Work out the finished part from the listing and answer in its coordinate system (mm). A direction names the side the tool comes from. Round coordinates to 2 decimals unless told otherwise and drop trailing zeros. Write each loop counter-clockwise with the first axis right and the second up, starting at its lowest first coordinate (ties: lowest second). Pieces come first, ordered by that corner, then holes.
from build123d import *

# Parameters (mm, degrees)
SKETCH_1_R          = 10
SKETCH_1_R_2        = 6
EXTRUDE_2_DEPTH     = 13
SKETCH_2_OUTSIDE_W  = 28.226
SKETCH_2_OUTSIDE_H  = 28.226
SKETCH_2_OUTSIDE_R  = 8.5
CUT_EXTRUDE_1_DEPTH = 9
CHAMFER_1_SIZE      = 0.5


with BuildPart() as part:
    # 草图1 → 凸台-拉伸2 (new body)
    with BuildSketch(Plane(origin=(0, 0, 0), x_dir=(0, 0, -1), z_dir=(1, 0, 0))):
        with Locations(Location((0, 0, 0), (0, 0, 180))):
            Circle(SKETCH_1_R)
        with Locations(Location((0, 0, 0), (0, 0, 180))):
            Circle(SKETCH_1_R_2, mode=Mode.SUBTRACT)
    extrude(amount=EXTRUDE_2_DEPTH)

    # 草图2 outside → 切除-拉伸1 (cut)
    with BuildSketch(Plane(origin=(13, 0, 0), x_dir=(0, 0, -1), z_dir=(1, 0, 0))):
        Rectangle(SKETCH_2_OUTSIDE_W, SKETCH_2_OUTSIDE_H)
        Circle(SKETCH_2_OUTSIDE_R, mode=Mode.SUBTRACT)
    extrude(amount=-CUT_EXTRUDE_1_DEPTH, mode=Mode.SUBTRACT)

    # 倒角1
    chamfer_1_edges = [part.edges().sort_by_distance(p)[0] for p in [
        (4, 0, -10),
        (13, 0, 8.5),
        (0, 0, -10),
        (0, 0, -6),
    ]]
    chamfer(chamfer_1_edges, length=CHAMFER_1_SIZE)


solid = part.part
Q1. Find section C-C (x = 9). Determine the outline of the cut face in (y, z).
Q2. Find the intervals of material crossed by L1, parallel to Y at x = 8.5, z = 0; L2, parallel to Y at x = 5, z = 5.25; L3, parallel to Z at x = 5.25, y = -2.75, in increasing order.
Q3. A tool of negligible diameter and unlimited length cuts with its end or side. For faces 4 (the face through (8.31, 7.167, -4.57)), 5 (the face through (13, -6, -2)), from which of +Z, -Z, +X, -X, +Y, -Y can it reach the whole face along a straight path? Write none if from no direction.
Q4. The mould has two halves that part along Y. Classify faces 1 (the face through (4, -8.4, 2.2)), 2 (the face through (2, 0, -10)), 3 (the face through (6.662, -1.802, 5.723)): +Y half, -Y half, draft (parallel to the pull), parting line (faces both ways), or undercut.
Q5. Find section A-A (y = 0). Determine the outline of the cut face in (x, z).
Q6. Given pin 1 (1.5 mm diameter, centred on y = 3.5, z = 3, fed in from -X); pin 2 (2 mm diameter, centred on x = 6, z = -3.5, fed in from -Y); pin 3 (5 mm diameter, centred on x = 7, y = 0, fed in from -Z); pin 4 (5 mm diameter, centred on x = 10, z = -3.5, fed in from -Y), each flat-ended and moving along its own axis, determine where each tip first touches the part or whether it passes through.
Report:
1. outline: circle Ø17 at (0, 0); hole circle Ø12 at (0, 0)
2. L1: y = -8.5 to -6, 6 to 8.5
2. L2: y = -6.68 to -2.9, 2.9 to 6.68
2. L3: z = -8.04 to -5.33, 5.33 to 8.04
3. face 4: +X
3. face 5: +Z, -Z, +X, +Y, -Y
4. face 1: draft
4. face 2: parting line
4. face 3: undercut
5. outline: (0, -9.5) - (0.5, -10) - (3.5, -10) - (4, -9.5) - (4, -8.5) - (12.5, -8.5) - (13, -8) - (13, -6) - (0.5, -6) - (0, -6.5) - close; (0, 6.5) - (0.5, 6) - (13, 6) - (13, 8) - (12.5, 8.5) - (4, 8.5) - (4, 9.5) - (3.5, 10) - (0.5, 10) - (0, 9.5) - close
6. pin 1: passes through
6. pin 2: stops at y = -8.12
6. pin 3: stops at z = -8.5
6. pin 4: stops at y = -8.44
